```python
from build123d import *

# Parameters (mm, degrees)
CROQUIS1_W              = 142
CROQUIS1_H              = 20.7
SALIENTE_EXTRUIR2_DEPTH = 3
CROQUIS6_R              = 1.5
CORTAR_EXTRUIR4_DEPTH   = 3
CROQUIS7_W              = 142
CROQUIS7_H              = 2
SALIENTE_EXTRUIR3_DEPTH = 9.7
CORTAR_EXTRUIR5_DEPTH   = 224
CROQUIS10_W             = 16.7
CROQUIS10_H             = 9.7
CORTAR_EXTRUIR6_DEPTH   = 80


with BuildPart() as part:
    # Croquis1 → Saliente-Extruir2 (new body)
    with BuildSketch(Plane(origin=(0, 0, 0), x_dir=(1, 0, 0), z_dir=(0, 1, 0))):
        Rectangle(CROQUIS1_W, CROQUIS1_H)
    extrude(amount=SALIENTE_EXTRUIR2_DEPTH)

    # Croquis6 → Cortar-Extruir4 (cut)
    with BuildSketch(Plane(origin=(0, 3, 0), x_dir=(1, 0, 0), z_dir=(0, 1, 0))):
        with Locations((-56, 0)):
            Circle(CROQUIS6_R)
        Circle(CROQUIS6_R)
        with Locations((56, 0)):
            Circle(CROQUIS6_R)
    extrude(amount=-CORTAR_EXTRUIR4_DEPTH, mode=Mode.SUBTRACT)

    # Croquis7 → Saliente-Extruir3 (add)
    with BuildSketch(Plane(origin=(0, 3, 0), x_dir=(1, 0, 0), z_dir=(0, 1, 0))):
        with Locations((0, 9.35)):
            Rectangle(CROQUIS7_W, CROQUIS7_H)
        with Locations((0, -9.35)):
            Rectangle(CROQUIS7_W, CROQUIS7_H)
    extrude(amount=SALIENTE_EXTRUIR3_DEPTH)

    # Croquis9 → Cortar-Extruir5 (cut)
    with BuildSketch(Plane.ZY.offset(71)):
        Polygon((-10.35, 2.7), (-9.85, 2.7), (-10.35, 1.2), align=None)
        Polygon((10.35, 2.7), (9.85, 2.7), (10.35, 1.2), align=None)
    extrude(amount=-CORTAR_EXTRUIR5_DEPTH, mode=Mode.SUBTRACT)

    # Croquis10 → Cortar-Extruir6 (cut)
    with BuildSketch(Plane.XY.offset(10.35)):
        with Locations((0, 7.85)):
            Rectangle(CROQUIS10_W, CROQUIS10_H)
    extrude(amount=-CORTAR_EXTRUIR6_DEPTH, mode=Mode.SUBTRACT)


solid = part.part
```
Verification items for the finished model (mm, model axes). A direction names the side the tool comes from. Round coordinates to 2 decimals unless told otherwise and drop trailing zeros. Write each loop counter-clockwise with the first axis right and the second up, starting at its lowest first coordinate (ties: lowest second). Pieces come first, ordered by that corner, then holes. Notation, with made-up numbers: (57, -24) -> (71, -24) arc R31 ccw to (71, 11) -> close; hole circle Ø2 at (68.25, -33). An arc over 180 degrees is marked (long way). Write each question's results on one line, items separated by ' | '. Start each with the question number.
1. Cross-section at C-C (x = 56). Enter the section's corners in (y, z).
2. Draft check along X on faces 1 (the flat face through (71, 2, 0)), 2 (the cylindrical face through (-54.57, 1.52, -0.45)), 3 (the flat face through (-1, 0, -2)), 4 (the flat face through (-71, 2, 0)). Enter one of: +X half, -X half, draft (parallel to the pull), parting line (faces both ways), or undercut.
3. Material ranges on probe 1 along X at (y, z) = (1.75, 0); probe 2 along Z at (x, y) = (-59.5, 5.75); probe 3 along Z at (x, y) = (-56, 0.95), recorded low to high. Write a range as from..to.
4. Depth check by flat-ended pin: P1, Ø1.8, axis at x = 56, z = 0, coming from the +Y side; P2, Ø8, axis at x = 46, z = -4, coming from the +Y side. Enter the tip coordinate at first touch or a pass-through.
5. Cross-section at A-A (z = 0). Enter the section's corners in (x, y), then the cut area to 3 significant figures.
6. Cross-section at B-B (y = 11). Enter the section's corners in (x, z), then the cut area to 3 significant figures.
7. Cross-section at D-D (x = 0). Enter the section's corners in (y, z), then the cut area to 4 significant figures.
8. Set-up check for faces 5 (the flat face through (-17, 8, -10.35)), 6 (the flat face through (39, 8, -8.35)): record each of +Z, -Z, +X, -X, +Y, -Y from which the full face is reachable in a straight line by a thin tool's end or side.
Solutions:
1) outline: (0, -10.35) -> (1.2, -10.35) -> (2.7, -9.85) -> (2.7, -10.35) -> (12.7, -10.35) -> (12.7, -8.35) -> (3, -8.35) -> (3, -1.5) -> (0, -1.5) -> close; (0, 1.5) -> (3, 1.5) -> (3, 8.35) -> (12.7, 8.35) -> (12.7, 10.35) -> (2.7, 10.35) -> (2.7, 9.85) -> (1.2, 10.35) -> (0, 10.35) -> close
2) face 1: +X half | face 2: undercut | face 3: draft | face 4: -X half
3) probe 1: x = -71..-57.5, -54.5..-1.5, 1.5..54.5, 57.5..71 | probe 2: z = -10.35..-8.35, 8.35..10.35 | probe 3: z = -10.35..-1.5, 1.5..10.35
4) P1: passes through | P2: stops at y = 3
5) outline: (-71, 0) -> (-57.5, 0) -> (-57.5, 3) -> (-71, 3) -> close; (-54.5, 0) -> (-1.5, 0) -> (-1.5, 3) -> (-54.5, 3) -> close; (1.5, 0) -> (54.5, 0) -> (54.5, 3) -> (1.5, 3) -> close; (57.5, 0) -> (71, 0) -> (71, 3) -> (57.5, 3) -> close | area: 399 mm2
6) outline: (-71, -10.35) -> (-8.35, -10.35) -> (-8.35, -8.35) -> (-71, -8.35) -> close; (-71, 8.35) -> (-8.35, 8.35) -> (-8.35, 10.35) -> (-71, 10.35) -> close; (8.35, -10.35) -> (71, -10.35) -> (71, -8.35) -> (8.35, -8.35) -> close; (8.35, 8.35) -> (71, 8.35) -> (71, 10.35) -> (8.35, 10.35) -> close | area: 501 mm2
7) outline: (0, -10.35) -> (1.2, -10.35) -> (2.7, -9.85) -> (2.7, -10.35) -> (3, -10.35) -> (3, -1.5) -> (0, -1.5) -> close; (0, 1.5) -> (3, 1.5) -> (3, 10.35) -> (2.7, 10.35) -> (2.7, 9.85) -> (1.2, 10.35) -> (0, 10.35) -> close | area: 52.35 mm2
8) face 5: -Z, +X, -X, +Y, -Y | face 6: +X, -X, +Y
